Geometry check sheet. Reference: the model listing, model coordinates, mm. A direction names the side the tool comes from. Give positions to 0.01 mm unless a question says otherwise; leave off trailing zeros. Write each loop counter-clockwise with the first axis right and the second up, starting at its lowest first coordinate (ties: lowest second). Pieces come first, ordered by that corner, then holes.
(1) Tool access check on faces 1 (the flat face through (9, 1.5, 0)), 2 (the cylindrical face through (-7.845, 0.74, -6.727)). Record the directions out of +Z, -Z, +X, -X, +Y, -Y that give a thin tool (end or side, any length) a straight path to the whole face; none if there is none.
(2) Cross-section at A-A (z = 3). Record the boundary of the cut face in (x, y).
(3) Cross-section at B-B (x = 2.25). Record the boundary of the cut face in (y, z), and give its area (3 significant figures).
(4) Mould release check, pull along X, two halves, no side actions. Record for faces 3 (the flat face through (0, 1, -10)), 4 (the cylindrical face through (-9.43, 0.74, -9.4)), 5 (the flat face through (-7, 1, -7.25)): +X half, -X half, draft (parallel to the pull), parting line (faces both ways), or undercut.
(5) Thickness scan on line 1 along X through (y, z) = (1, -1.5); line 2 along Z through (x, y) = (5.25, 0.1). Record the ranges inside material, lowest first.
(6) Depth check by flat-ended pin: P1, Ø3, axis at x = -6.5, z = 1, coming from the +Y side. Enter the tip coordinate at first touch or a pass-through.
Autodesk Inventor part; units mm, degrees
ref_plane "YZ Plane" through (0, 0, 0) normal (1, 0, 0) x (0, 1, 0)
ref_plane "XZ Plane" through (0, 0, 0) normal (0, 1, 0) x (-1, 0, 0)
ref_plane "XY Plane" through (0, 0, 0) normal (0, 0, 1) x (1, 0, 0)
sketch "Sketch1" plane through (0, 0, 0) normal (0, 1, 0) x (-1, 0, 0)
  line L0 (7.25, 5.8376) -> (7.25, -5.8376)
  line L1 (-7.25, -5.8376) -> (-7.25, 5.8376)
  line L2 (-7.25, 7.25) -> (7.25, -7.25) construction
  line L3 (7.25, 7.25) -> (-7.25, -7.25) construction
  line L4 (6.25, 7.25) -> (2.75, 7.25) construction
  line L5 (2.75, 7.35) -> (2.75, 7.95)
  line L6 (3.25, 8.45) -> (5.75, 8.45)
  line L7 (6.25, 7.95) -> (6.25, 7.35)
  arc A0 (7.4265, 6.0765) -> (7.25, 7.25) centre (7.25, 6.65) ccw
  line L8 (-7.25, 7.25) -> (2.65, 7.25)
  line L9 (6.35, 7.25) -> (7.25, 7.25)
  arc A1 (6.25, 7.35) -> (6.35, 7.25) centre (6.35, 7.35) ccw
  arc A2 (2.65, 7.25) -> (2.75, 7.35) centre (2.65, 7.35) ccw
  arc A3 (6.25, 7.95) -> (5.75, 8.45) centre (5.75, 7.95) ccw
  arc A4 (3.25, 8.45) -> (2.75, 7.95) centre (3.25, 7.95) ccw
  arc A5 (7.4265, 6.0765) -> (7.25, 5.8376) centre (7.5, 5.8376) ccw
  line L10 (0, 0) -> (2.8942, 0)
  line L11 (0, 0) -> (0, -4.9214)
  line L12 (7.25, -7.25) -> (-7.25, 7.25) construction
  line L13 (6.25, -7.25) -> (2.75, -7.25) construction
  line L14 (2.75, -7.35) -> (2.75, -7.95)
  line L15 (3.25, -8.45) -> (5.75, -8.45)
  line L16 (6.25, -7.95) -> (6.25, -7.35)
  arc A6 (7.25, -7.25) -> (7.4265, -6.0765) centre (7.25, -6.65) ccw
  line L17 (6.35, -7.25) -> (7.25, -7.25)
  arc A7 (6.35, -7.25) -> (6.25, -7.35) centre (6.35, -7.35) ccw
  arc A8 (2.75, -7.35) -> (2.65, -7.25) centre (2.65, -7.35) ccw
  arc A9 (5.75, -8.45) -> (6.25, -7.95) centre (5.75, -7.95) ccw
  arc A10 (2.75, -7.95) -> (3.25, -8.45) centre (3.25, -7.95) ccw
  arc A11 (7.25, -5.8376) -> (7.4265, -6.0765) centre (7.5, -5.8376) ccw
  line L18 (7.25, -7.25) -> (6.35, -7.25)
  line L19 (-6.25, 7.25) -> (-2.75, 7.25) construction
  line L20 (-2.75, 7.35) -> (-2.75, 7.95)
  line L21 (-3.25, 8.45) -> (-5.75, 8.45)
  line L22 (-6.25, 7.95) -> (-6.25, 7.35)
  arc A12 (-7.25, 7.25) -> (-7.4265, 6.0765) centre (-7.25, 6.65) ccw
  line L23 (-6.35, 7.25) -> (-7.25, 7.25)
  arc A13 (-6.35, 7.25) -> (-6.25, 7.35) centre (-6.35, 7.35) ccw
  arc A14 (-2.75, 7.35) -> (-2.65, 7.25) centre (-2.65, 7.35) ccw
  arc A15 (-5.75, 8.45) -> (-6.25, 7.95) centre (-5.75, 7.95) ccw
  arc A16 (-2.75, 7.95) -> (-3.25, 8.45) centre (-3.25, 7.95) ccw
  arc A17 (-7.25, 5.8376) -> (-7.4265, 6.0765) centre (-7.5, 5.8376) ccw
  arc A18 (-7.4265, -6.0765) -> (-7.25, -5.8376) centre (-7.5, -5.8376) ccw
  arc A19 (-7.4265, -6.0765) -> (-7.25, -7.25) centre (-7.25, -6.65) ccw
  line L24 (-6.35, -7.25) -> (-7.25, -7.25)
  line L25 (-7.25, -7.25) -> (7.25, 7.25) construction
  arc A20 (-6.25, -7.35) -> (-6.35, -7.25) centre (-6.35, -7.35) ccw
  line L26 (-6.25, -7.95) -> (-6.25, -7.35)
  arc A21 (-6.25, -7.95) -> (-5.75, -8.45) centre (-5.75, -7.95) ccw
  line L27 (-6.25, -7.25) -> (-2.75, -7.25) construction
  line L28 (-3.25, -8.45) -> (-5.75, -8.45)
  arc A22 (-2.65, -7.25) -> (-2.75, -7.35) centre (-2.65, -7.35) ccw
  line L29 (-2.75, -7.35) -> (-2.75, -7.95)
  arc A23 (-3.25, -8.45) -> (-2.75, -7.95) centre (-3.25, -7.95) ccw
  line L30 (-7.25, -7.25) -> (-6.35, -7.25)
  line L31 (2.65, -7.25) -> (-2.65, -7.25)
  line L32 (-6.35, -7.25) -> (-7.25, -7.25)
  line L33 (8, -10) -> (-8, -10)
  line L34 (-10, -8) -> (-10, 8)
  line L35 (-8, 10) -> (8, 10)
  line L36 (10, 8) -> (10, -8)
  arc A24 (10, 8) -> (8, 10) centre (8, 8) ccw
  arc A25 (8, -10) -> (10, -8) centre (8, -8) ccw
  arc A26 (-10, -8) -> (-8, -10) centre (-8, -8) ccw
  arc A27 (-8, 10) -> (-10, 8) centre (-8, 8) ccw
  point P0 (2.75, 8.45)
  point P1 (6.25, 8.45)
  point P2 (6.25, 7.65)
  point P3 (7.25, 6.05)
  point P4 (2.75, -8.45)
  point P5 (6.25, -8.45)
  point P6 (6.25, -7.65)
  point P7 (7.25, -6.05)
  point P8 (-2.75, 8.45)
  point P9 (-6.25, 8.45)
  point P10 (-6.25, 7.65)
  point P11 (-7.25, 6.05)
  point P12 (-7.25, -6.05)
  point P13 (-6.25, -7.65)
  point P14 (-6.25, -8.45)
  point P15 (-2.75, -8.45)
  point P16 (10, -10)
  point P17 (-10, -10)
  point P18 (-10, 10)
  point P19 (10, 10)
  point P20 (-7.25, 7.25)
  point P21 (-6.35, 7.25)
  point P22 (-2.65, 7.25)
  dimension "d0" = 14.5
  dimension "d1" = 14.5
  dimension "d2" = 3.5
  dimension "d3" = 1.2
  dimension "d4" = 1
  dimension "d5" = 1.2
  dimension "d6" = 0.1
  dimension "d7" = 0.1
  dimension "d8" = 0.5
  dimension "d9" = 0.25
  dimension "d10" = 2
  dimension "d13" = 20
  dimension "d14" = 20
extrude "Extrusion1" add sketch "Sketch1" along normal blind 1.5
properties part number "test switch hole"
Reply:
1. face 1: +Z, -Z, +X, -X, +Y
1. face 2: +Y, -Y
2. outline: (-10, 0) - (-7.25, 0) - (-7.25, 1.5) - (-10, 1.5) - close; (7.25, 0) - (10, 0) - (10, 1.5) - (7.25, 1.5) - close
3. outline: (0, -10) - (1.5, -10) - (1.5, -7.25) - (0, -7.25) - close; (0, 7.25) - (1.5, 7.25) - (1.5, 10) - (0, 10) - close
3. area: 8.25 mm2
4. face 3: draft
4. face 4: -X half
4. face 5: undercut
5. line 1: x = -10 to -7.25, 7.25 to 10
5. line 2: z = -10 to -8.45, 8.45 to 10
6. P1: stops at y = 1.5
